Source: CAD feature listing. Evaluate the final solid. Frame: model axes, mm. A direction names the side the tool comes from. Round coordinates to 2 decimals unless told otherwise and drop trailing zeros. Order: outer loops, then holes, each group sorted by start corner. A loop starts at its lowest first (then second) coordinate and runs counter-clockwise, first axis right, second up. Notation, with made-up numbers: (77.5, -22.5) -> (114.5, -22.5) arc R8 ccw to (114.5, -11.5) -> close; hole circle Ø6 at (65, 63.5). An arc over 180 degrees is marked (long way). Answer as CSV lines item,"result". Start each with the question number.
(1) Section query A-A (y = 11.25). Output: boundary loops of the cut face in (x, z).
(2) Set-up query: faces 5 (the cylindrical face through (7.07, 2.85, -5.01)), 6 (the cylindrical face through (-8.958, 5.804, -7.711)), 7 (the flat face through (9, 13, 6)), 8 (the cylindrical face through (9.042, 5.804, -7.711)), 9 (the flat face through (0, 12, -11)). Return all of +Z, -Z, +X, -X, +Y, -Y with unobstructed straight access to the full face (end or side cutting, diameter ignored); none if empty.
(3) Contact query for flat-ended pins moving along their axis: P1, Ø1.5, axis at x = -3, z = 6, coming from the -Y side; P2, Ø2, axis at x = -0.5, z = 9.5, coming from the -Y side; P3, Ø1, axis at x = -7, y = 10.5, coming from the +Z side; P4, Ø3.5, axis at x = 8, z = 0, coming from the -Y side. Output: stop coordinate, or through.
(4) Pull-direction query (Z, two-part tool) for faces 1 (the flat face through (-7, 11, -2)), 2 (the cylindrical face through (-8.958, 5.711, 7.804)), 3 (the flat face through (6, 10, -9)), 4 (the cylindrical face through (6, 14, 0)); classes: +Z half, -Z half, draft (parallel to the pull), parting line (faces both ways), or undercut.
(5) Line query: line 1 along Z through (x, y) = (0, 14.05); line 2 along X through (y, z) = (9.25, 3). Output: solid intervals per line, ascending. Write a range as from..to.
(6) Section query C-C (x = -7.25). Output: boundary loops of the cut face in (y, z).
(7) Section query D-D (z = -7). Output: boundary loops of the cut face in (x, y).
(8) Section query B-B (z = 0). Output: boundary loops of the cut face in (x, y).
```python
from build123d import *

# Parameters (mm, degrees)
EXTRUDE_1_DEPTH     = 12
CUT_EXTRUDE_5_DEPTH = 24
EXTRUDE_5_DEPTH     = 24
SKETCH_2_4_W        = 4
SKETCH_2_4_H        = 12
CUT_EXTRUDE_6_DEPTH = 12
SKETCH_9_R          = 2
CUT_EXTRUDE_7_DEPTH = 4


with BuildPart() as part:
    # Sketch 2 → Extrude 1 (new, symmetric)
    with BuildSketch(Plane.XY):
        Polygon((-2, 0), (-12, 0), (-12, 4), (-6, 4), (-6, 16), (6, 16), (6, 4), (12, 4), (12, 0), (2, 0), (2, 12), (-2, 12), align=None)
    extrude(amount=EXTRUDE_1_DEPTH, both=True)

    # Sketch 7 → Cut-Extrude 5 (cut)
    with BuildSketch(Plane(origin=(12, 0, 0), x_dir=(0, 0, -1), z_dir=(1, 0, 0))):
        with BuildLine():
            Line((-12, 0), (12, 0))
            ThreePointArc((12, 0), (4.928932188, 2.928932188), (2, 10))
            Line((2, 10), (2, 12))
            Line((2, 12), (-2, 12))
            Line((-2, 12), (-2, 10))
            ThreePointArc((-2, 10), (-4.928932188, 2.928932188), (-12, 0))
        make_face()
    extrude(amount=-CUT_EXTRUDE_5_DEPTH, mode=Mode.SUBTRACT)

    # Sketch 7_4 → Extrude 5 (add)
    with BuildSketch(Plane(origin=(12, 0, 0), x_dir=(0, 0, -1), z_dir=(1, 0, 0))):
        with BuildLine():
            ThreePointArc((12, 0), (4.928932188, 2.928932188), (2, 10))
            Line((2, 10), (2, 12))
            Line((2, 12), (-2, 12))
            Line((-2, 12), (-2, 10))
            ThreePointArc((-2, 10), (-4.928932188, 2.928932188), (-12, 0))
            Line((-12, 0), (-12, 4))
            ThreePointArc((-12, 4), (-7.757359313, 5.757359313), (-6, 10))
            Line((-6, 10), (-6, 16))
            Line((-6, 16), (6, 16))
            Line((6, 16), (6, 10))
            ThreePointArc((6, 10), (7.757359313, 5.757359313), (12, 4))
            Line((12, 4), (12, 0))
        make_face()
    extrude(amount=-EXTRUDE_5_DEPTH)

    # Sketch 2_4 → Cut-Extrude 6 (cut, symmetric)
    with BuildSketch(Plane.XY):
        with Locations((0, 6)):
            Rectangle(SKETCH_2_4_W, SKETCH_2_4_H)
    extrude(amount=CUT_EXTRUDE_6_DEPTH, both=True, mode=Mode.SUBTRACT)

    # Sketch 9 → Cut-Extrude 7 (cut)
    with BuildSketch(Plane(origin=(0, 16, 0), x_dir=(1, 0, 0), z_dir=(0, 1, 0))):
        with Locations(Location((0, 8, 0), (0, 0, 270))):
            Circle(SKETCH_9_R)
        with Locations(Location((-8, 0, 0), (0, 0, 270))):
            Circle(SKETCH_9_R)
        with Locations(Location((8, 0, 0), (0, 0, 90))):
            Circle(SKETCH_9_R)
        with Locations(Location((0, -8, 0), (0, 0, 180))):
            Circle(SKETCH_9_R)
    extrude(amount=-CUT_EXTRUDE_7_DEPTH, mode=Mode.SUBTRACT)


solid = part.part
```
Answer block:
1,outline,"(-12, -6) -> (-6, -6) -> (-6, -12) -> (-2, -12) -> (-2, -2) -> (-12, -2) -> close; (-12, 2) -> (-2, 2) -> (-2, 12) -> (-6, 12) -> (-6, 6) -> (-12, 6) -> close; (2, -12) -> (6, -12) -> (6, -6) -> (12, -6) -> (12, -2) -> (2, -2) -> close; (2, 2) -> (12, 2) -> (12, 6) -> (6, 6) -> (6, 12) -> (2, 12) -> close"
2,face 5,"+X, -X, -Y"
2,face 6,"-Z, -X, +Y"
2,face 7,"+Z, +X, +Y"
2,face 8,"-Z, +X, +Y"
2,face 9,"+Z, -Z, -Y"
3,P1,"y = 1.49"
3,P2,"y = 12"
3,P3,"z = 6"
3,P4,"through"
4,face 1,"undercut"
4,face 2,"+Z half"
4,face 3,"draft"
4,face 4,"undercut"
5,line 1,"-12..-10, -6..6, 10..12"
5,line 2,"-12..-2, 2..12"
6,outline,"(0, -12) -> (4, -12) arc R6 cw to (10, -6) -> (16, -6) -> (16, -1.85) -> (12, -1.85) -> (12, -2) -> (10, -2) arc R10 ccw to start; (0, 12) arc R10 ccw to (10, 2) -> (12, 2) -> (12, 1.85) -> (16, 1.85) -> (16, 6) -> (10, 6) arc R6 cw to (4, 12) -> close"
7,outline,"(-12, 1.34) -> (-2, 1.34) -> (-2, 12) -> (-1.73, 12) -> (-1.73, 16) -> (-6, 16) -> (-6, 6.68) -> (-12, 6.68) -> close; (1.73, 12) -> (2, 12) -> (2, 1.34) -> (12, 1.34) -> (12, 6.68) -> (6, 6.68) -> (6, 16) -> (1.73, 16) -> close"
8,outline,"(-12, 12) -> (-10, 12) -> (-10, 16) -> (-12, 16) -> close; (-6, 12) -> (6, 12) -> (6, 16) -> (-6, 16) -> close; (10, 12) -> (12, 12) -> (12, 16) -> (10, 16) -> close"
